Work out the finished part from the listing and answer in its coordinate system (mm). Face numbers are marked on the shaded views. Coordinates: 2 decimals unless noted, no trailing zeros. Write each loop counter-clockwise with the first axis right and the second up, starting at its lowest first coordinate (ties: lowest second). Pieces come first, ordered by that corner, then holes. Notation, with made-up numbers: M 56,-9 L 65,-9 A10 ccw 65,4 Z; hole C -7,33 d1. An arc over 180 degrees is marked long. Answer as CSV lines item,"result". Start each with the question number.
(1) The mould has two halves that part along Y. Classify the marked faces 1, 2 and 3: released by +Y, released by -Y, zero draft, split by the parting line, or undercut.
(2) A cutting plane is placed at A-A on x = 0. Give the vertices of the cut face in (y, z), then the cut area to 3 significant figures.
(3) Flat-ended cylindrical pins translate along their axes: P1, Ø1, axis at x = 9.5, z = 5, coming from the +Y side; P2, Ø3, axis at y = -15, z = 5, coming from the -X side. Find the tip coordinate at first contact, or state that the pin passes through.
(4) A cutting plane is placed at C-C on x = -15. Give the vertices of the cut face in (y, z).
(5) Find the intervals of material crossed by L1, parallel to Y at x = 0, z = 1.5; L2, parallel to X at y = 0.5, z = 1.5; L3, parallel to X at y = -1, z = 4.75, in increasing order. Write a range as [from, to].
from build123d import *

# Parameters (mm, degrees)
SKETCH1_R             = 22.5
SKETCH1_R_2           = 4
SKETCH1_R_3           = 1.89865
SKETCH1_R_4           = 1.9939
BOSS_EXTRUDE1_DEPTH   = 6.35
CHAMFER1_SIZE         = 2.301024407
CHAMFER1_SIZE2        = 2.00025
CHAMFER1_PART_2_SIZE  = 2.301024407
CHAMFER1_PART_2_SIZE2 = 2.00025
CHAMFER1_PART_3_SIZE  = 2.301024407
CHAMFER1_PART_3_SIZE2 = 2.00025
CHAMFER1_PART_4_SIZE  = 2.301024407
CHAMFER1_PART_4_SIZE2 = 2.00025


with BuildPart() as part:
    # Sketch1 → Boss-Extrude1 (new body)
    with BuildSketch(Plane.XY):
        Circle(SKETCH1_R)
        Circle(SKETCH1_R_2, mode=Mode.SUBTRACT)
        with Locations((0, 15)):
            Circle(SKETCH1_R_3, mode=Mode.SUBTRACT)
        with Locations((10.606601718, 10.606601718)):
            Circle(SKETCH1_R_4, mode=Mode.SUBTRACT)
        with Locations((15, 0)):
            Circle(SKETCH1_R_3, mode=Mode.SUBTRACT)
        with Locations((10.606601718, -10.606601718)):
            Circle(SKETCH1_R_4, mode=Mode.SUBTRACT)
        with Locations((0, -15)):
            Circle(SKETCH1_R_3, mode=Mode.SUBTRACT)
        with Locations((-10.606601718, -10.606601718)):
            Circle(SKETCH1_R_4, mode=Mode.SUBTRACT)
        with Locations((-15, 0)):
            Circle(SKETCH1_R_3, mode=Mode.SUBTRACT)
        with Locations((-10.606601718, 10.606601718)):
            Circle(SKETCH1_R_4, mode=Mode.SUBTRACT)
    extrude(amount=BOSS_EXTRUDE1_DEPTH)

    # Chamfer1
    chamfer1_edges = [part.edges().sort_by_distance(p)[0] for p in [
        (13.10135, 0, 6.35),
    ]]
    chamfer1_side = [part.faces().sort_by_distance(p)[0] for p in [
        (13.10135, 0, 3.175),
    ]]
    chamfer(chamfer1_edges, length=CHAMFER1_SIZE, length2=CHAMFER1_SIZE2, reference=chamfer1_side[0])

    # Chamfer1 part 2
    chamfer1_part_2_edges = [part.edges().sort_by_distance(p)[0] for p in [
        (-1.89865, -15, 6.35),
    ]]
    chamfer1_part_2_side = [part.faces().sort_by_distance(p)[0] for p in [
        (-1.89865, -15, 3.175),
    ]]
    chamfer(chamfer1_part_2_edges, length=CHAMFER1_PART_2_SIZE, length2=CHAMFER1_PART_2_SIZE2, reference=chamfer1_part_2_side[0])

    # Chamfer1 part 3
    chamfer1_part_3_edges = [part.edges().sort_by_distance(p)[0] for p in [
        (-16.89865, 0, 6.35),
    ]]
    chamfer1_part_3_side = [part.faces().sort_by_distance(p)[0] for p in [
        (-16.89865, 0, 3.175),
    ]]
    chamfer(chamfer1_part_3_edges, length=CHAMFER1_PART_3_SIZE, length2=CHAMFER1_PART_3_SIZE2, reference=chamfer1_part_3_side[0])

    # Chamfer1 part 4
    chamfer1_part_4_edges = [part.edges().sort_by_distance(p)[0] for p in [
        (-1.89865, 15, 6.35),
    ]]
    chamfer1_part_4_side = [part.faces().sort_by_distance(p)[0] for p in [
        (-1.89865, 15, 3.175),
    ]]
    chamfer(chamfer1_part_4_edges, length=CHAMFER1_PART_4_SIZE, length2=CHAMFER1_PART_4_SIZE2, reference=chamfer1_part_4_side[0])


solid = part.part
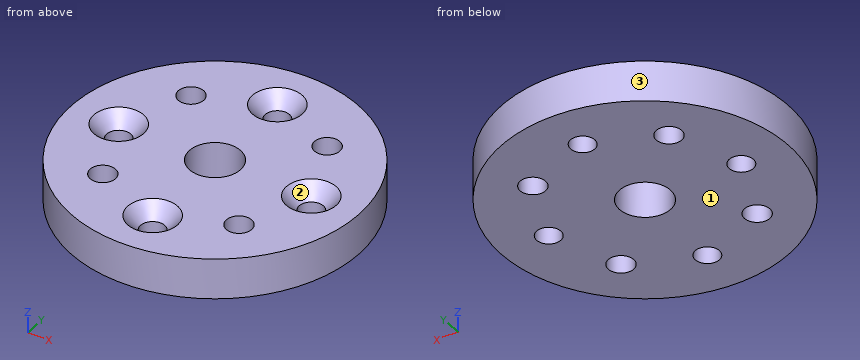
Here are the results:
1,face 1,"zero draft"
1,face 2,"undercut"
1,face 3,"split by the parting line"
2,outline,"M -22.5,0 L -16.9,0 L -16.9,4.05 L -18.9,6.35 L -22.5,6.35 Z; M -13.1,0 L -4,0 L -4,6.35 L -11.1,6.35 L -13.1,4.05 Z; M 4,0 L 13.1,0 L 13.1,4.05 L 11.1,6.35 L 4,6.35 Z; M 16.9,0 L 22.5,0 L 22.5,6.35 L 18.9,6.35 L 16.9,4.05 Z"
2,area,"178 mm^2"
3,P1,"stops at y = 20.62"
3,P2,"stops at x = -18"
4,outline,"M -16.77,0 L -1.9,0 L -1.9,4.05 L -3.9,6.35 L -16.77,6.35 Z; M 1.9,0 L 16.77,0 L 16.77,6.35 L 3.9,6.35 L 1.9,4.05 Z"
5,L1,"y = [-22.5, -16.9], [-13.1, -4], [4, 13.1], [16.9, 22.5]"
5,L2,"x = [-22.49, -16.83], [-13.17, -3.97], [3.97, 13.17], [16.83, 22.49]"
5,L3,"x = [-22.48, -17.3], [-12.7, -3.87], [3.87, 12.7], [17.3, 22.48]"
